```python
from build123d import *

# Parameters (mm, degrees)
SKETCH_1_R      = 1.05
SKETCH_1_W      = 8.5
SKETCH_1_H      = 8.5
EXTRUDE_1_DEPTH = 1.5
FILLET_1_R      = 1


with BuildPart() as part:
    # 草图1 → 凸台-拉伸1 (new body)
    with BuildSketch(Plane.XY):
        Polygon((1.45, 41.958612035), (27.19, 41.958612035), (27.19, 46.958612035), (24.99, 46.958612035), (24.99, 48.458612035), (29.39, 48.458612035), (29.39, 46.958612035), (28.69, 46.958612035), (28.69, 41.958612035), (33.69, 41.958612035), (33.69, 56.958612035), (14.32, 56.958612035), (-5.05, 56.958612035), (-5.05, 41.958612035), (-0.05, 41.958612035), (-0.05, 46.958612035), (-0.75, 46.958612035), (-0.75, 48.458612035), (3.65, 48.458612035), (3.65, 46.958612035), (1.45, 46.958612035), align=None)
        with Locations((27.94, 53.458612035)):
            Circle(SKETCH_1_R, mode=Mode.SUBTRACT)
        with Locations(Location((0.7, 53.458612035, 0), (0, 0, 180))):
            Circle(SKETCH_1_R, mode=Mode.SUBTRACT)
        with Locations((14.32, 51.458612035)):
            Rectangle(SKETCH_1_W, SKETCH_1_H, mode=Mode.SUBTRACT)
    extrude(amount=EXTRUDE_1_DEPTH)

    # 圆角1
    fillet_1_edges = [part.edges().sort_by_distance(p)[0] for p in [
        (-5.05, 41.958612035, 0.75),
        (-5.05, 56.958612035, 0.75),
        (33.69, 56.958612035, 0.75),
        (33.69, 41.958612035, 0.75),
    ]]
    fillet(fillet_1_edges, radius=FILLET_1_R)


solid = part.part
```
Work out the finished part from the listing and answer in its coordinate system (mm). A direction names the side the tool comes from. Give positions to 0.01 mm unless a question says otherwise; leave off trailing zeros. Order: outer loops, then holes, each group sorted by start corner. A loop starts at its lowest first (then second) coordinate and runs counter-clockwise, first axis right, second up. Notation, with made-up numbers: M -18.5,-33 L 33.5,-33 A17 ccw 33.5,-16 Z; hole C 58.25,66 d8. An arc over 180 degrees is marked long. Return JSON: item names as keys, results as strings.
1) Straight lines are drawn through the part: line 1 along X through (y, z) = (44.5, 1.45); line 2 along X through (y, z) = (48.25, 0.1); line 3 along X through (y, z) = (47, 0.3). For each, find the intervals that lie inside material, in ascending order. Write a range as [from, to].
Resolved:
{"line 1": "[-5.05, -0.05], [1.45, 27.19], [28.69, 33.69]", "line 2": "[-5.05, -0.75], [3.65, 10.07], [18.57, 24.99], [29.39, 33.69]", "line 3": "[-5.05, -0.75], [3.65, 24.99], [29.39, 33.69]"}
2) This flat-tipped pin is pushed along its axis until it touches: pin 1 (1.3 mm diameter, centred on x = 27.94, y = 53.46, fed in from -Z). Where does it stop, or does it pass through?
Resolved:
{"pin 1": "through"}
3) Section A-A, the plane x = 0.7 is taken. Write down the section's boundary in (y, z).
Resolved:
{"outline": "M 48.46,0 L 52.41,0 L 52.41,1.5 L 48.46,1.5 Z; M 54.51,0 L 56.96,0 L 56.96,1.5 L 54.51,1.5 Z"}
4) Section C-C, the plane y = 47.75 is taken. Write down the section's boundary in (x, z).
Resolved:
{"outline": "M -5.05,0 L -0.75,0 L -0.75,1.5 L -5.05,1.5 Z; M 3.65,0 L 10.07,0 L 10.07,1.5 L 3.65,1.5 Z; M 18.57,0 L 24.99,0 L 24.99,1.5 L 18.57,1.5 Z; M 29.39,0 L 33.69,0 L 33.69,1.5 L 29.39,1.5 Z"}
5) Section B-B, the plane y = 44 is taken. Write down the section's boundary in (x, z).
Resolved:
{"outline": "M -5.05,0 L -0.05,0 L -0.05,1.5 L -5.05,1.5 Z; M 1.45,0 L 27.19,0 L 27.19,1.5 L 1.45,1.5 Z; M 28.69,0 L 33.69,0 L 33.69,1.5 L 28.69,1.5 Z"}
6) For a pull along X with two mould halves and no side action, classify faces 4 (the flat face through (27.19, 44, 1)), 5 (the flat face through (-5.05, 50, 1)), 6 (the flat face through (15, 56.959, 1)) as +X half, -X half, draft (parallel to the pull), parting line (faces both ways), or undercut.
Resolved:
{"face 4": "undercut", "face 5": "-X half", "face 6": "draft"}
7) A tool of negligible diameter and unlimited length cuts with its end or side. For faces 1 (the flat face through (28.69, 44, 1)), 2 (the flat face through (10.07, 51, 1)), 3 (the cylindrical face through (-4.76, 56.66, 0.76)), from which of +Z, -Z, +X, -X, +Y, -Y can it reach the whole face along a straight path? Write none if from no direction.
Resolved:
{"face 1": "+Z, -Z, -Y", "face 2": "+Z, -Z", "face 3": "+Z, -Z, -X, +Y"}
8) Section D-D, the plane z = 0.3 is taken. Give the number of separate pieces and of enclosed holes in the cut face, plus the area to 3 significant figures.
Resolved:
{"separate pieces": "1", "enclosed holes": "3", "area": "473 mm^2"}
